Geometry check sheet. Reference: drawing and pictorial views, mm from the part's lowest x, y, z. Give positions to 0.01 mm unless a question says otherwise; leave off trailing zeros. Loops run counter-clockwise (first coordinate to the right, second up) from the corner with the lowest first, then second, coordinate; pieces in that order, holes last. Notation, with made-up numbers: (68.5, -22) -> (110.5, -22) arc R34 cw to (110.5, 16) -> close; hole circle Ø6 at (-38.5, 17.25). An arc over 180 degrees is marked (long way). Write each question's results on one line, items separated by ' | '. Start each with the question number.
1. Cross-section at A-A on y = 1.95. Count the separate pieces of the cut face and the enclosed holes in it, and give its area (3 significant figures).
2. Cross-section at B-B on x = 60. Record the boundary of the cut face in (y, z).
3. Material ranges on L1, parallel to X at y = 3, z = 60; L2, parallel to X at y = 1.75, z = 51 (1 decimal); L3, parallel to X at y = 1.2, z = 60, recorded low to high. Write a range as from..to.
4. Cross-section at D-D on x = 45. Record the boundary of the cut face in (y, z) (1 decimal), and give its area (3 significant figures).
5. Cross-section at C-C on z = 60. Record the boundary of the cut face in (x, y).
6. Gauge pin test, flat ends, axial feed: pin 1 Ø24 at (x, z) = (74.5, 61.5) entering from +Y; pin 2 Ø2 at (x, y) = (75, 3) entering from +Z; pin 3 Ø16 at (x, z) = (60, 60) entering from +Y; pin 4 Ø1.5 at (y, z) = (3, 56.5) entering from -X. Record the tip position at first contact, or that the pin passes through.
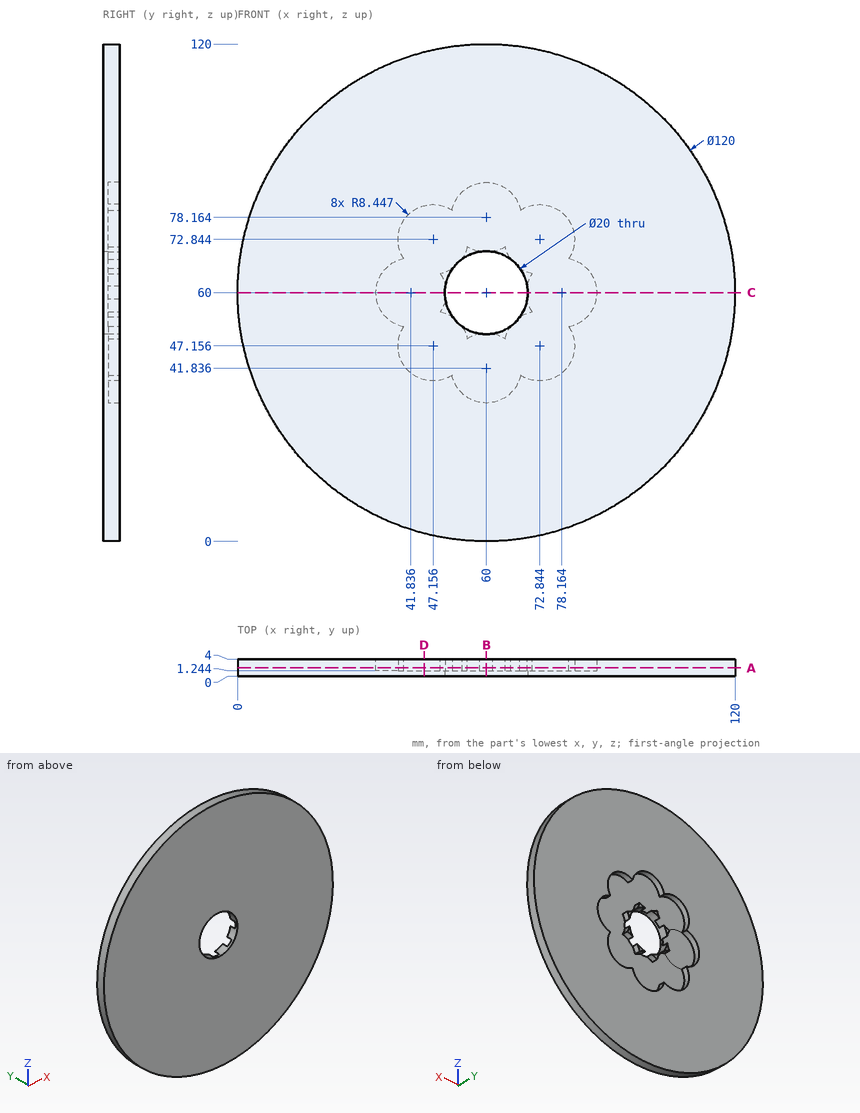
Geometry says:
1) separate pieces: 9 | enclosed holes: 1 | area: 9,360 mm^2
2) outline: (0, 0) -> (4, 0) -> (4, 33.39) -> (1.24, 33.39) -> (1.24, 50) -> (0, 50) -> close; (0, 70) -> (1.24, 70) -> (1.24, 86.61) -> (4, 86.61) -> (4, 120) -> (0, 120) -> close
3) L1: 0..33.39, 86.61..120 | L2: 0.7..39.6, 54.7..55.6, 64.4..65.3, 80.4..119.3 | L3: 0..50, 70..120
4) outline: (0, 1.9) -> (4, 1.9) -> (4, 39) -> (1.2, 39) -> (1.2, 81) -> (4, 81) -> (4, 118.1) -> (0, 118.1) -> close | area: 349 mm^2
5) outline: (0, 0) -> (50, 0) -> (50, 1.24) -> (33.39, 1.24) -> (33.39, 4) -> (0, 4) -> close; (70, 0) -> (120, 0) -> (120, 4) -> (86.61, 4) -> (86.61, 1.24) -> (70, 1.24) -> close
6) pin 1: y = 4 | pin 2: z = 118.34 | pin 3: through | pin 4: x = 0.06
